from build123d import *

# Parameters (mm, degrees)
SALIENTE_EXTRUIR1_DEPTH = 4
CROQUIS2_R              = 1.7
CORTAR_EXTRUIR1_DEPTH   = 4
CROQUIS3_R              = 2.95
CORTAR_EXTRUIR2_DEPTH   = 3


with BuildPart() as part:
    # Croquis1 → Saliente-Extruir1 (new body)
    with BuildSketch(Plane.XY):
        with BuildLine():
            Line((-7.200520814, -3.25), (-15, -3.25))
            Line((-15, -3.25), (-15, 3.25))
            Line((-15, 3.25), (-7.200520814, 3.25))
            ThreePointArc((-7.200520814, 3.25), (0, 7.9), (7.200520814, 3.25))
            Line((7.200520814, 3.25), (15, 3.25))
            Line((15, 3.25), (15, -3.25))
            Line((15, -3.25), (7.200520814, -3.25))
            ThreePointArc((7.200520814, -3.25), (0, -7.9), (-7.200520814, -3.25))
        make_face()
    extrude(amount=SALIENTE_EXTRUIR1_DEPTH)

    # Croquis2 → Cortar-Extruir1 (cut)
    with BuildSketch(Plane.XY.offset(4)):
        with Locations((-11, 0)):
            Circle(CROQUIS2_R)
        with Locations((11, 0)):
            Circle(CROQUIS2_R)
    extrude(amount=-CORTAR_EXTRUIR1_DEPTH, mode=Mode.SUBTRACT)

    # Croquis3 → Cortar-Extruir2 (cut)
    with BuildSketch(Plane.XY.offset(4)):
        with Locations((-11, 0)):
            Circle(CROQUIS3_R)
        with Locations((11, 0)):
            Circle(CROQUIS3_R)
    extrude(amount=-CORTAR_EXTRUIR2_DEPTH, mode=Mode.SUBTRACT)


solid = part.part
Source: CAD feature listing. Evaluate the final solid. Frame: model axes, mm. A direction names the side the tool comes from. Round coordinates to 2 decimals unless told otherwise and drop trailing zeros. Loops run counter-clockwise (first coordinate to the right, second up) from the corner with the lowest first, then second, coordinate; pieces in that order, holes last.
Q1. Section C-C, the plane y = 0. Return loops of the section in (x, z), plus the area to 3 significant figures.
Q2. Mould query, pull axis X, two halves, no side actions, for faces 5 (the face through (-0.1, 7.9, 2)), 6 (the face through (-11, -3.25, 2)), 7 (the face through (12.57, -0.65, 0.51)). Classes: pulls with the +X half, pulls with the -X half, needs draft (parallel to the pull), parting line crosses it, or undercut.
Q3. Section D-D, the plane z = 2.8. Return loops of the section in (x, y), plus the area to 3 significant figures.
Q4. First-contact query: P1, Ø1.5, axis at x = 9.5, z = 3, coming from the -Y side; P2, Ø2.5, axis at x = -11, y = 0, coming from the -Z side; P3, Ø2, axis at x = 11.5, z = 2, coming from the +Y side; P4, Ø1.5, axis at x = -3.5, z = 2.5, coming from the -Y side. Flat tips, straight axial feed; report the tip coordinate or a pass-through.
Q5. Ray query, line 1 (Y direction, x = -11, z = 0.45); line 2 (Y direction, x = -11, z = 2.85); line 3 (X direction, y = 2, z = 3.5). Return the intervals inside material, ascending.
Q6. Section B-B, the plane z = 0.45. Return loops of the section in (x, y).
Q7. Access query for faces 1 (the face through (11, 3.25, 2)), 2 (the face through (-11, 3.25, 2)), 3 (the face through (11, -3.25, 2)), 4 (the face through (8.053, 0.13, 2.521)). Directions: +Z, -Z, +X, -X, +Y, -Y. A direction counts if a zero-diameter tool reaches every point of the face in a straight line with its end or side. Return the directions, or none.
Q8. Section A-A, the plane x = 11. Return loops of the section in (y, z), plus the area to 3 significant figures.
Solutions:
1. outline: (-15, 0) - (-12.7, 0) - (-12.7, 1) - (-13.95, 1) - (-13.95, 4) - (-15, 4) - close; (-9.3, 0) - (9.3, 0) - (9.3, 1) - (8.05, 1) - (8.05, 4) - (-8.05, 4) - (-8.05, 1) - (-9.3, 1) - close; (12.7, 0) - (15, 0) - (15, 4) - (13.95, 4) - (13.95, 1) - (12.7, 1) - close
1. area: 77.8 mm2
2. face 5: parting line crosses it
2. face 6: needs draft
2. face 7: undercut
3. outline: (-15, -3.25) - (-7.2, -3.25) arc R7.9 ccw to (7.2, -3.25) - (15, -3.25) - (15, 3.25) - (7.2, 3.25) arc R7.9 ccw to (-7.2, 3.25) - (-15, 3.25) - close; hole circle Ø5.9 at (-11, 0); hole circle Ø5.9 at (11, 0)
3. area: 237 mm2
4. P1: stops at y = -3.25
4. P2: passes through
4. P3: stops at y = 3.25
4. P4: stops at y = -7.41
5. line 1: y = -3.25 to -1.7, 1.7 to 3.25
5. line 2: y = -3.25 to -2.95, 2.95 to 3.25
5. line 3: x = -15 to -13.17, -8.83 to 8.83, 13.17 to 15
6. outline: (-15, -3.25) - (-7.2, -3.25) arc R7.9 ccw to (7.2, -3.25) - (15, -3.25) - (15, 3.25) - (7.2, 3.25) arc R7.9 ccw to (-7.2, 3.25) - (-15, 3.25) - close; hole circle Ø3.4 at (-11, 0); hole circle Ø3.4 at (11, 0)
7. face 1: +Z, -Z, +X, +Y
7. face 2: +Z, -Z, -X, +Y
7. face 3: +Z, -Z, +X, -Y
7. face 4: +Z
8. outline: (-3.25, 0) - (-1.7, 0) - (-1.7, 1) - (-2.95, 1) - (-2.95, 4) - (-3.25, 4) - close; (1.7, 0) - (3.25, 0) - (3.25, 4) - (2.95, 4) - (2.95, 1) - (1.7, 1) - close
8. area: 4.90 mm2
